Geometry check sheet. Reference: the model listing, model coordinates, mm. A direction names the side the tool comes from. Round coordinates to 2 decimals unless told otherwise and drop trailing zeros. Order: outer loops, then holes, each group sorted by start corner. A loop starts at its lowest first (then second) coordinate and runs counter-clockwise, first axis right, second up. Notation, with made-up numbers: (55, 65.5) - (65, 65.5) arc R16 cw to (65, 93.5) - close; hole circle Ø2 at (47, 58). An arc over 180 degrees is marked (long way). Return JSON: item names as keys, results as strings. Group by question number.
Q1. Sectioned sample at D-D, the plane y = -6. Record the cut outline in (x, z), then the cut area to 3 significant figures.
Q2. Gauge pin test, flat ends, axial feed: pin 1 Ø0.6 at (x, y) = (21.5, -29.5) entering from +Z; pin 2 Ø2 at (x, y) = (10.5, -29.5) entering from -Z; pin 3 Ø0.6 at (x, y) = (-1, -15.5) entering from -Z. Record the tip position at first contact, or that the pin passes through.
Q3. Tool access check on faces 4 (the flat face through (23, -29, 2)), 5 (the flat face through (33, -18.25, 21)), 6 (the flat face through (9, -29, 9)), 7 (the flat face through (21, -28, 10)). Record the directions out of +Z, -Z, +X, -X, +Y, -Y that give a thin tool (end or side, any length) a straight path to the whole face; none if there is none.
Q4. Sectioned sample at C-C, the plane z = 14.5. Record the cut outline in (x, y), then the cut area to 3 significant figures.
Q5. Sectioned sample at B-B, the plane z = 8.5. Record the cut outline in (x, y), then the cut area to 3 significant figures.
Q6. Material ranges on line 1 along Y through (x, z) = (38, 18); line 2 along X through (y, z) = (-13, 13); line 3 along Z through (x, y) = (17.5, -9), recorded low to high.
Q7. Sectioned sample at A-A, the plane y = -11.5. Record the cut outline in (x, z).
Q8. Draft check along X on faces 1 (the flat face through (20, -14, 22)), 2 (the cylindrical face through (43.1, -29.14, 9.13)), 3 (the flat face through (6, -29, 4)). Enter one of: pulls with the +X half, pulls with the -X half, needs draft (parallel to the pull), parting line crosses it, or undercut.
```python
from build123d import *

# Parameters (mm, degrees)
SKETCH1_W                = 46
SKETCH1_H                = 32
SKETCH1_W_2              = 42
SKETCH1_H_2              = 28
BOSS_EXTRUDE1_DEPTH      = 20
SKETCH2_W                = 46
SKETCH2_H                = 32
BOSS_EXTRUDE2_DEPTH      = 2
SKETCH3_W                = 8
SKETCH3_H                = 4
CUT_EXTRUDE2_DEPTH       = 58.965506985
SKETCH4_W                = 5
SKETCH4_H                = 5
CUT_EXTRUDE3_DEPTH       = 2
SKETCH5_W                = 46
SKETCH5_H                = 32
BOSS_EXTRUDE3_DEPTH      = 2
SKETCH6_W                = 8.5
SKETCH6_H                = 4.25
CUT_EXTRUDE4_DEPTH       = 2
SKETCH7_W                = 11.5
SKETCH7_H                = 11.5
SKETCH7_W_2              = 8.5
SKETCH7_H_2              = 8.5
BOSS_EXTRUDE5_DEPTH      = 2
SKETCH9_R                = 5.75
SKETCH9_R_2              = 5
BOSS_EXTRUDE8_DEPTH      = 4
BOSS_EXTRUDE9_DEPTH      = 0.5
FILLET2_R                = 4
FILLET3_R                = 3
FILLET4_R                = 2
SKETCH13_W               = 43
SKETCH13_H               = 32
CUT_EXTRUDE5_DEPTH       = 2
SKETCH14_W               = 2
SKETCH14_H               = 32
CUT_EXTRUDE6_DEPTH       = 2
SKETCH15_W               = 4
SKETCH15_H               = 4
CUT_EXTRUDE9_DEPTH       = 2
SKETCH16_W               = 1.236067977
SKETCH16_H               = 30.472135954
CUT_EXTRUDE10_DEPTH      = 2
FILLET9_R                = 3
CUT_EXTRUDE11_DEPTH      = 62.188234163
CUT_EXTRUDE11_DEPTH_BACK = 62.188234163
SKETCH19_W               = 4
SKETCH19_H               = 2
SKETCH21_W               = 2
SKETCH21_H               = 4
CUT_EXTRUDE12_DEPTH      = 55
SKETCH22_W               = 4
SKETCH22_H               = 4
BOSS_EXTRUDE10_DEPTH     = 2
SKETCH23_W               = 4
SKETCH23_H               = 4
BOSS_EXTRUDE11_DEPTH     = 2
SKETCH24_W               = 6
SKETCH24_H               = 5
CUT_EXTRUDE13_DEPTH      = 46.5
SKETCH25_W               = 5
SKETCH25_H               = 10
CUT_EXTRUDE14_DEPTH      = 13
CUT_EXTRUDE15_START      = -3.5
SKETCH26_R               = 6.5
SKETCH26_R_2             = 5
CUT_EXTRUDE15_DEPTH      = 3.5
SKETCH27_W               = 11.5
SKETCH27_H               = 11.5
CUT_EXTRUDE16_DEPTH      = 2.5


with BuildPart() as part:
    # Sketch1 → Boss-Extrude1 (new body)
    with BuildSketch(Plane.XY):
        with Locations((21, -14)):
            Rectangle(SKETCH1_W, SKETCH1_H)
        with Locations((21, -14)):
            Rectangle(SKETCH1_W_2, SKETCH1_H_2, mode=Mode.SUBTRACT)
    extrude(amount=BOSS_EXTRUDE1_DEPTH)

    # Sketch2 → Boss-Extrude2 (add)
    with BuildSketch(Plane(origin=(0, 0, 0), x_dir=(-1, 0, 0), z_dir=(0, 0, -1))):
        with Locations((-21, -14)):
            Rectangle(SKETCH2_W, SKETCH2_H)
    extrude(amount=BOSS_EXTRUDE2_DEPTH)

    # Sketch3 → Cut-Extrude2 (cut, through all)
    with BuildSketch(Plane.XZ.offset(30)):
        with Locations((6, 2)):
            Rectangle(SKETCH3_W, SKETCH3_H)
    extrude(amount=-CUT_EXTRUDE2_DEPTH, mode=Mode.SUBTRACT)

    # Sketch4 → Cut-Extrude3 (cut)
    with BuildSketch(Plane.ZY.offset(2)):
        with Locations((2.5, -11.5)):
            Rectangle(SKETCH4_W, SKETCH4_H)
        with Locations((2.5, -16.5)):
            Rectangle(SKETCH4_W, SKETCH4_H)
    extrude(amount=-CUT_EXTRUDE3_DEPTH, mode=Mode.SUBTRACT)

    # Sketch5 → Boss-Extrude3 (add)
    with BuildSketch(Plane.XY.offset(20)):
        with Locations((21, -14)):
            Rectangle(SKETCH5_W, SKETCH5_H)
    extrude(amount=BOSS_EXTRUDE3_DEPTH)

    # Sketch6 → Cut-Extrude4 (cut)
    with BuildSketch(Plane.XY.offset(22)):
        with Locations((32.75, -11.875)):
            Rectangle(SKETCH6_W, SKETCH6_H)
        with Locations((32.75, -16.125)):
            Rectangle(SKETCH6_W, SKETCH6_H)
    extrude(amount=-CUT_EXTRUDE4_DEPTH, mode=Mode.SUBTRACT)

    # Sketch7 → Boss-Extrude5 (add)
    with BuildSketch(Plane.XY.offset(22)):
        with Locations((32.75, -14)):
            Rectangle(SKETCH7_W, SKETCH7_H)
        with Locations((32.75, -14)):
            Rectangle(SKETCH7_W_2, SKETCH7_H_2, mode=Mode.SUBTRACT)
    extrude(amount=BOSS_EXTRUDE5_DEPTH)

    # Sketch9 → Boss-Extrude8 (add)
    with BuildSketch(Plane.XY.offset(24)):
        with Locations((32.75, -14)):
            Circle(SKETCH9_R)
        with Locations(Location((32.75, -14, 0), (0, 0, 211.788330617))):
            Circle(SKETCH9_R_2, mode=Mode.SUBTRACT)
    extrude(amount=BOSS_EXTRUDE8_DEPTH)

    # Sketch11 → Boss-Extrude9 (add)
    with BuildSketch(Plane.XY.offset(24)):
        with BuildLine():
            Line((38.5, -19.75), (38.5, -14))
            ThreePointArc((38.5, -14), (38.111902647, -16.076655966), (37, -17.872983346))
            Line((37, -17.872983346), (37, -18.25))
            Line((37, -18.25), (36.622983346, -18.25))
            ThreePointArc((36.622983346, -18.25), (34.826655966, -19.361902647), (32.75, -19.75))
            Line((32.75, -19.75), (38.5, -19.75))
        make_face()
        with BuildLine():
            Line((27, -19.75), (29.718911087, -19.75))
            ThreePointArc((29.718911087, -19.75), (28.153805922, -18.596194078), (27, -17.031088913))
            Line((27, -17.031088913), (27, -19.75))
        make_face()
        with BuildLine():
            Line((38.5, -10.968911087), (38.5, -8.25))
            Line((38.5, -8.25), (35.781088913, -8.25))
            ThreePointArc((35.781088913, -8.25), (37.346194078, -9.403805922), (38.5, -10.968911087))
        make_face()
        with BuildLine():
            Line((27, -8.25), (27, -10.968911087))
            ThreePointArc((27, -10.968911087), (28.153805922, -9.403805922), (29.718911087, -8.25))
            Line((29.718911087, -8.25), (27, -8.25))
        make_face()
    extrude(amount=BOSS_EXTRUDE9_DEPTH)

    # Fillet2
    fillet2_edges = [part.edges().sort_by_distance(p)[0] for p in [
        (44, -14, 22),
    ]]
    fillet(fillet2_edges, radius=FILLET2_R)

    # Fillet3
    fillet3_edges = [part.edges().sort_by_distance(p)[0] for p in [
        (19, 2, 22),
        (44, 2, 8),
        (42.828427125, 2, 20.828427125),
        (44, -30, 8),
        (42.828427125, -30, 20.828427125),
        (44, -14, -2),
        (19, -30, 22),
    ]]
    fillet(fillet3_edges, radius=FILLET3_R)

    # Fillet4
    fillet4_edges = [part.edges().sort_by_distance(p)[0] for p in [
        (27, -8.25, 23.25),
        (27, -19.75, 23.25),
        (38.5, -19.75, 23.25),
        (38.5, -8.25, 23.25),
    ]]
    fillet(fillet4_edges, radius=FILLET4_R)

    # Sketch13 → Cut-Extrude5 (cut)
    with BuildSketch(Plane(origin=(0, 0, -2), x_dir=(-1, 0, 0), z_dir=(0, 0, -1))):
        with Locations((-19.5, -14)):
            Rectangle(SKETCH13_W, SKETCH13_H)
    extrude(amount=-CUT_EXTRUDE5_DEPTH, mode=Mode.SUBTRACT)

    # Sketch14 → Cut-Extrude6 (cut)
    with BuildSketch(Plane.ZY.offset(-41)):
        with Locations((-1, -14)):
            Rectangle(SKETCH14_W, SKETCH14_H)
    extrude(amount=-CUT_EXTRUDE6_DEPTH, mode=Mode.SUBTRACT)

    # Sketch15 → Cut-Extrude9 (cut)
    with BuildSketch(Plane.XY.offset(22)):
        with Locations((13, -25)):
            Rectangle(SKETCH15_W, SKETCH15_H)
    extrude(amount=-CUT_EXTRUDE9_DEPTH, mode=Mode.SUBTRACT)

    # Sketch16 → Cut-Extrude10 (cut)
    with BuildSketch(Plane.ZY.offset(-43)):
        with Locations((-0.618033989, -14)):
            Rectangle(SKETCH16_W, SKETCH16_H)
    extrude(amount=-CUT_EXTRUDE10_DEPTH, mode=Mode.SUBTRACT)

    # Fillet9
    fillet9_edges = [part.edges().sort_by_distance(p)[0] for p in [
        (-2, -14, 22),
        (-2, -30, 9.5),
        (-2, 2, 9.5),
        (-2, 1.121320344, 21.121320344),
        (-2, -29.121320344, 21.121320344),
    ]]
    fillet(fillet9_edges, radius=FILLET9_R)

    # Sketch19 → Cut-Extrude11 (cut, two sides: drawn at the far end of the back side and taken through both)
    with BuildSketch(Plane.XZ.offset(30).offset(-CUT_EXTRUDE11_DEPTH_BACK)):
        with Locations((21, 2.5)):
            Rectangle(SKETCH19_W, SKETCH19_H)
    extrude(amount=CUT_EXTRUDE11_DEPTH + CUT_EXTRUDE11_DEPTH_BACK, mode=Mode.SUBTRACT)

    # Sketch21 → Cut-Extrude12 (cut, symmetric)
    with BuildSketch(Plane(origin=(0, 2, 0), x_dir=(1, 0, 0), z_dir=(0, 1, 0))):
        with Locations((11, -2)):
            Rectangle(SKETCH21_W, SKETCH21_H)
    extrude(amount=CUT_EXTRUDE12_DEPTH, both=True, mode=Mode.SUBTRACT)

    # Sketch22 → Boss-Extrude10 (add)
    with BuildSketch(Plane(origin=(0, 2, 0), x_dir=(1, 0, 0), z_dir=(0, 1, 0))):
        with Locations((4, -2)):
            Rectangle(SKETCH22_W, SKETCH22_H)
    extrude(amount=-BOSS_EXTRUDE10_DEPTH)

    # Sketch23 → Boss-Extrude11 (add)
    with BuildSketch(Plane.XZ.offset(30)):
        with Locations((4, 2)):
            Rectangle(SKETCH23_W, SKETCH23_H)
    extrude(amount=-BOSS_EXTRUDE11_DEPTH)

    # Sketch24 → Cut-Extrude13 (cut, symmetric)
    with BuildSketch(Plane.XZ.offset(30)):
        with Locations((9, 6.5)):
            Rectangle(SKETCH24_W, SKETCH24_H)
    extrude(amount=CUT_EXTRUDE13_DEPTH, both=True, mode=Mode.SUBTRACT)

    # Sketch25 → Cut-Extrude14 (cut)
    with BuildSketch(Plane.ZY.offset(2)):
        with Locations((7.5, -14)):
            Rectangle(SKETCH25_W, SKETCH25_H)
    extrude(amount=-CUT_EXTRUDE14_DEPTH, mode=Mode.SUBTRACT)

    # Sketch26 → Cut-Extrude15 (cut)
    with BuildSketch(Plane.XY.offset(28).offset(CUT_EXTRUDE15_START)):
        with Locations((32.75, -14)):
            Circle(SKETCH26_R)
        with Locations(Location((32.75, -14, 0), (0, 0, 211.788330617))):
            Circle(SKETCH26_R_2, mode=Mode.SUBTRACT)
    extrude(amount=CUT_EXTRUDE15_DEPTH, mode=Mode.SUBTRACT)

    # Sketch27 → Cut-Extrude16 (cut)
    with BuildSketch(Plane.XY.offset(24.5)):
        with Locations((32.75, -14)):
            Rectangle(SKETCH27_W, SKETCH27_H)
    extrude(amount=-CUT_EXTRUDE16_DEPTH, mode=Mode.SUBTRACT)


solid = part.part
```
Reply:
{
 "1": {"outline": "(-2, 0) - (0, 0) - (0, 20) - (42, 20) - (42, 0) - (43.83, 0) arc R3 ccw to (44, 1) - (44, 18) arc R4 ccw to (40, 22) - (1, 22) arc R3 ccw to (-2, 19) - close", "area": "167 mm^2"},
 "2": {"pin 1": "z = 21.04", "pin 2": "z = 9", "pin 3": "z = 10"},
 "3": {"face 4": "+Y, -Y", "face 5": "+Z, -Z", "face 6": "-Z, +Y, -Y", "face 7": "-Z"},
 "4": {"outline": "(-2, -27) arc R3 ccw to (1, -30) - (41, -30) arc R3 ccw to (44, -27) - (44, -1) arc R3 ccw to (41, 2) - (1, 2) arc R3 ccw to (-2, -1) - close; hole (0, -28) - (42, -28) - (42, 0) - (0, 0) - close", "area": "288 mm^2"},
 "5": {"outline": "(-2, -27) arc R3 ccw to (1, -30) - (6, -30) - (6, -28) - (0, -28) - (0, -19) - (-2, -19) - close; (-2, -9) - (0, -9) - (0, 0) - (6, 0) - (6, 2) - (1, 2) arc R3 ccw to (-2, -1) - close; (12, -30) - (41, -30) arc R3 ccw to (44, -27) - (44, -1) arc R3 ccw to (41, 2) - (12, 2) - (12, 0) - (42, 0) - (42, -28) - (12, -28) - close", "area": "244 mm^2"},
 "6": {"line 1": "-30 to -28, 0 to 2", "line 2": "-2 to 0, 42 to 44", "line 3": "20 to 22"},
 "7": {"outline": "(-2, 10) - (0, 10) - (0, 20) - (28.5, 20) - (28.5, 22) - (1, 22) arc R3 ccw to (-2, 19) - close; (37, 20) - (42, 20) - (42, 0) - (43.83, 0) arc R3 ccw to (44, 1) - (44, 18) arc R4 ccw to (40, 22) - (37, 22) - close"},
 "8": {"face 1": "needs draft", "face 2": "pulls with the +X half", "face 3": "undercut"}
}
